Autodesk Inventor part; units mm, degrees
ref_plane "YZ Plane" through (0, 0, 0) normal (1, 0, 0) x (0, 1, 0)
ref_plane "XZ Plane" through (0, 0, 0) normal (0, 1, 0) x (-1, 0, 0)
ref_plane "XY Plane" through (0, 0, 0) normal (0, 0, 1) x (1, 0, 0)
sketch "Sketch1" plane through (0, 0, 0) normal (0, 1, 0) x (-1, 0, 0)
  line L0 (50, 0) -> (-50, 0)
  line L1 (0, 50) -> (0, -50)
  line L2 (-25.0156, 15.5413) -> (-25.0156, -28.4587)
  arc A0 (-25.0156, -28.4587) -> (-18.8156, -34.6587) centre (-18.8156, -28.4587) ccw
  line L3 (-18.8156, -34.6587) -> (25.1844, -34.6587)
  arc A1 (25.1844, -34.6587) -> (31.3844, -28.4587) centre (25.1844, -28.4587) ccw
  line L4 (31.3844, -28.4587) -> (31.3844, 15.5413)
  line L5 (31.3844, 15.5413) -> (37.1483, 89.6103)
  arc A2 (37.1483, 89.6103) -> (16.2805, 98.5862) centre (25.1844, 90.5413) ccw
  line L6 (16.2805, 98.5862) -> (0.0171, 80.5862)
  arc A3 (0.0171, 80.5862) -> (-25.0156, 15.5413) centre (72.0072, 15.5413) ccw
  line L7 (31.3844, 15.5413) -> (-25.0156, 15.5413) construction
  point P0 (0, 0)
  point P1 (31.3844, 15.5413)
  dimension "d0" = 100
  dimension "d1" = 100
  dimension "d3" = 56.4
  dimension "d4" = 6.2
  dimension "case_foot_outer_radius" = 12
  dimension "case_foot_width" = 75
  dimension "d7" = 18
extrude "Extrusion1" add sketch "Sketch1" along normal blind 1
equation "\"d3\" = core_outer_width + 2 * case_spacing + 2 * case_thickness"
equation "\"d4\" = core_outer_radius + case_thickness + case_spacing"
equation "\"case_spacing\" = 0.2"
properties part number "m2stack_bottom_1"
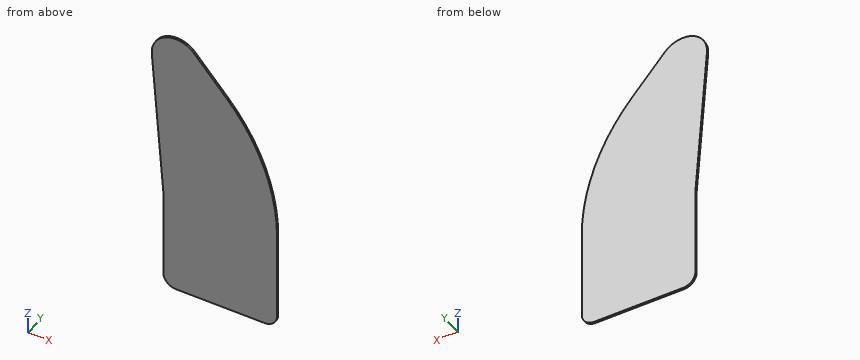
Design review of the part built by this model. Coordinates are the model's own, in mm. Coordinates: 2 decimals unless noted, no trailing zeros. Order: outer loops, then holes, each group sorted by start corner. A loop starts at its lowest first (then second) coordinate and runs counter-clockwise, first axis right, second up. Notation, with made-up numbers: (83.25, 15) -> (94.25, 15) arc R28 ccw to (94.25, 37) -> close; hole circle Ø2 at (71, -32.75). An arc over 180 degrees is marked (long way). One line per item, written item: value.
1) To check wall thickness, follow probe 1 along X at (y, z) = (0.5, 15); probe 2 along X at (y, z) = (0.4, 60); probe 3 along Z at (x, y) = (16.5, 0.4). State the ranges of each line that lie inside material, in increasing order. Write a range as [from, to].
Output values:
probe 1: x = [-31.38, 25.02]
probe 2: x = [-34.84, 14.23]
probe 3: z = [-34.66, 55.29]
2) We need section A-A, the plane y = 0.75. Give the boundary of the cut face in (x, z), then the cut area to 3 significant figures.
Output values:
outline: (-37.15, 89.61) -> (-31.38, 15.54) -> (-31.38, -28.46) arc R6.2 ccw to (-25.18, -34.66) -> (18.82, -34.66) arc R6.2 ccw to (25.02, -28.46) -> (25.02, 15.54) arc R97.02 ccw to (-0.02, 80.59) -> (-16.28, 98.59) arc R12 ccw to start
area: 6,700 mm2
3) We need section C-C, the plane x = -9. Give the boundary of the cut face in (y, z), then the cut area to 3 significant figures.
Output values:
outline: (0, -34.66) -> (1, -34.66) -> (1, 90.53) -> (0, 90.53) -> close
area: 125 mm2
4) We need section B-B, the plane z = -16. Give the boundary of the cut face in (x, y).
Output values:
outline: (-31.38, 0) -> (25.02, 0) -> (25.02, 1) -> (-31.38, 1) -> close
